Geometry: see drawing. Coordinates: mm, zero at the bounding-box minimum. A direction names the side the tool comes from. Round coordinates to 2 decimals unless told otherwise and drop trailing zeros. Order: outer loops, then holes, each group sorted by start corner. A loop starts at its lowest first (then second) coordinate and runs counter-clockwise, first axis right, second up. Notation, with made-up numbers: (38.5, -33) -> (57.5, -33) arc R21 cw to (57.5, -5) -> close; hole circle Ø4 at (8, 56.5). An arc over 180 degrees is marked (long way). Answer as CSV lines item,"result". Start each with the question number.
(1) Section query A-A (y = 29). Output: boundary loops of the cut face in (x, z).
(2) Line query: line 1 along X through (y, z) = (27, 27); line 2 along Y through (x, z) = (61.5, 21) (1 decimal); line 3 along X through (y, z) = (51.5, 10). Output: solid intervals per line, ascending. Write a range as from..to.
(3) Set-up query: the marked faces 4, 5 and 6. Return all of +Z, -Z, +X, -X, +Y, -Y with unobstructed straight access to the full face (end or side cutting, diameter ignored); none if empty.
(4) Contact query for flat-ended pins moving along their axis: P1, Ø5, axis at x = 27, y = 42, coming from the -Z side; P2, Ø4, axis at x = 34.5, y = 61, coming from the -Z side; P3, Ø10, axis at y = 57, z = 30.5, coming from the -X side; P4, Ø5, axis at x = 53.5, z = 7.5, coming from the +Y side. Output: stop coordinate, or through.
(5) Pull-direction query (X, two-part tool) for the marked faces 1, 2 and 3; classes: +X half, -X half, draft (parallel to the pull), parting line (faces both ways), or undercut.
(6) Section query C-C (y = 42). Output: boundary loops of the cut face in (x, z) (1 decimal).
(7) Section query D-D (x = 18). Output: boundary loops of the cut face in (y, z) (1 decimal).
(8) Section query B-B (z = 35.5). Output: boundary loops of the cut face in (x, y) (1 decimal), plus the area to 3 significant figures.
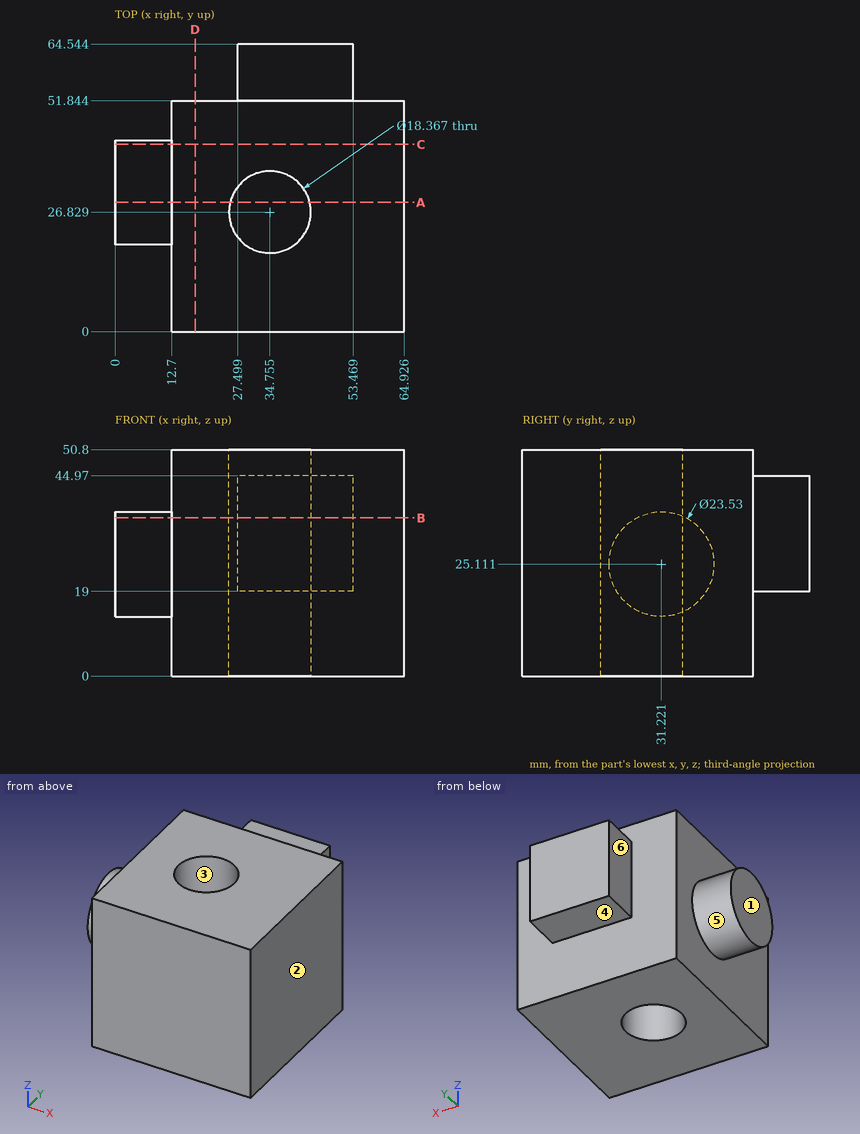
Answer block:
1,outline,"(0, 13.56) -> (12.7, 13.56) -> (12.7, 0) -> (25.83, 0) -> (25.83, 50.8) -> (12.7, 50.8) -> (12.7, 36.66) -> (0, 36.66) -> close; (43.68, 0) -> (64.93, 0) -> (64.93, 50.8) -> (43.68, 50.8) -> close"
2,line 1,"0..25.57, 43.94..64.93"
2,line 2,"0..51.8"
2,line 3,"12.7..64.93"
3,face 4,"-Z, +X, -X, +Y"
3,face 5,"-X"
3,face 6,"+Z, -Z, -X, +Y"
4,P1,"z = 0"
4,P2,"z = 19"
4,P3,"x = 27.5"
4,P4,"y = 51.84"
5,face 1,"-X half"
5,face 2,"+X half"
5,face 3,"undercut"
6,outline,"(0, 20.4) -> (12.7, 20.4) -> (12.7, 0) -> (64.9, 0) -> (64.9, 50.8) -> (12.7, 50.8) -> (12.7, 29.8) -> (0, 29.8) -> close"
7,outline,"(0, 0) -> (51.8, 0) -> (51.8, 50.8) -> (0, 50.8) -> close"
8,outline,"(0, 25.7) -> (12.7, 25.7) -> (12.7, 0) -> (64.9, 0) -> (64.9, 51.8) -> (53.5, 51.8) -> (53.5, 64.5) -> (27.5, 64.5) -> (27.5, 51.8) -> (12.7, 51.8) -> (12.7, 36.7) -> (0, 36.7) -> close; hole circle Ø18.4 at (34.8, 26.8)"
8,area,"2,910 mm2"
